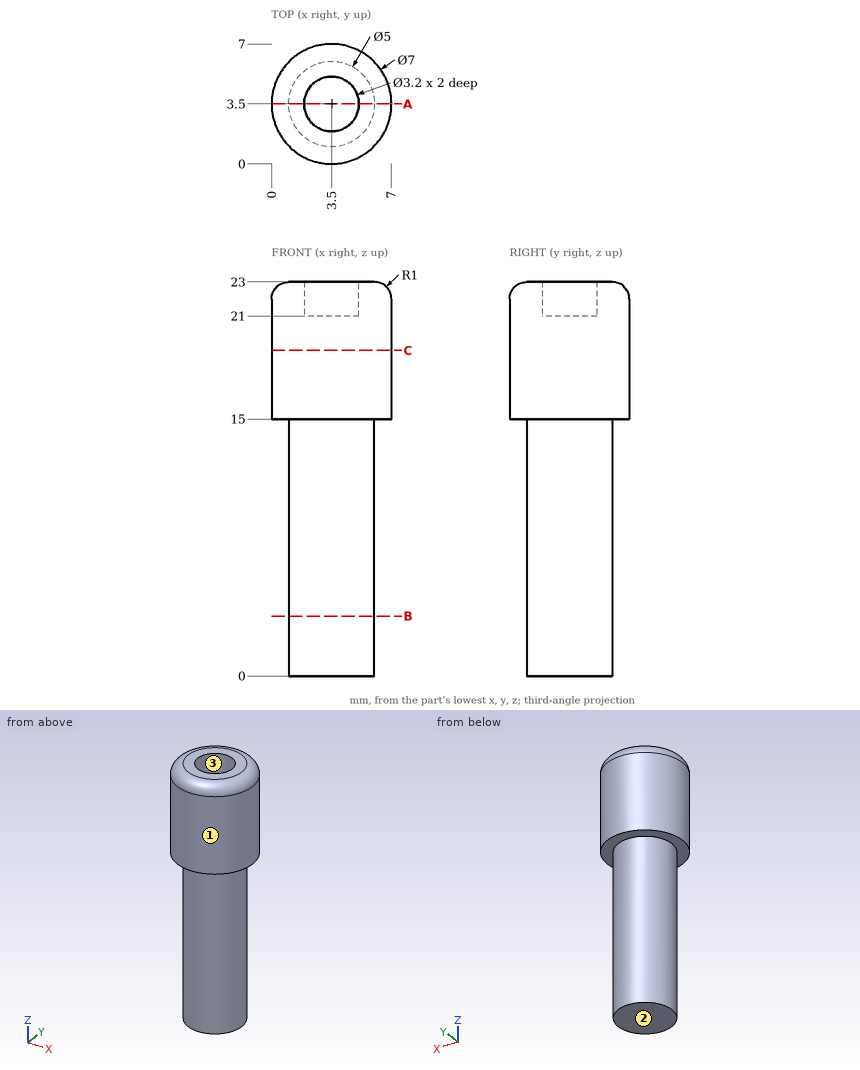
The figure shows three views and two pictorial views of one solid part (mm, origin at its lowest corner). Answer the questions. Round coordinates to 2 decimals unless told otherwise and drop trailing zeros. Order: outer loops, then holes, each group sorted by start corner. A loop starts at its lowest first (then second) coordinate and runs counter-clockwise, first axis right, second up. Notation, with made-up numbers: (89.5, 64.25) - (139.5, 64.25) arc R5 ccw to (139.5, 72.25) - close; hole circle Ø1 at (52, 30). An arc over 180 degrees is marked (long way). Write item = value, one per line. Start each with the question number.
1) Straight lines are drawn through the part: L1, parallel to Y at x = 3.5, z = 22.05; L2, parallel to Y at x = 3.5, z = 22.45; L3, parallel to Z at x = 4.5, y = 3.75. For each, find the intervals that lie inside material, in ascending order.
2) Section B-B, the plane z = 3.5 is taken. Write down the section's boundary in (x, y), plus the area to 3 significant figures.
3) Section A-A, the plane y = 3.5 is taken. Write down the section's boundary in (x, z), plus the area to 3 significant figures.
4) For a pull along X with two mould halves and no side action, classify the marked faces 1, 2 and 3 as released by +X, released by -X, zero draft, split by the parting line, or undercut.
5) Section C-C, the plane z = 19 is taken. Write down the section's boundary in (x, y), plus the area to 3 significant figures.
6) Given pin 1 (1 mm diameter, centred on x = 3, y = 4, fed in from +Z); pin 2 (1 mm diameter, centred on y = 3, z = 4.5, fed in from -X); pin 3 (2 mm diameter, centred on y = 5, z = 16, fed in from -X), each flat-ended and moving along its own axis, determine where each tip first touches the part or whether it passes through.
Results list:
q1.L1 = 0 to 1.9, 5.1 to 7
q1.L2 = 0.11 to 1.9, 5.1 to 6.89
q1.L3 = 0 to 21
q2.outline = circle Ø5 at (3.5, 3.5)
q2.area = 19.6 mm^2
q3.outline = (0, 15) - (1, 15) - (1, 0) - (6, 0) - (6, 15) - (7, 15) - (7, 22) arc R1 ccw to (6, 23) - (5.1, 23) - (5.1, 21) - (1.9, 21) - (1.9, 23) - (1, 23) arc R1 ccw to (0, 22) - close
q3.area = 124 mm^2
q4.face_1 = split by the parting line
q4.face_2 = zero draft
q4.face_3 = undercut
q5.outline = circle Ø7 at (3.5, 3.5)
q5.area = 38.5 mm^2
q6.pin_1 = 21
q6.pin_2 = 1
q6.pin_3 = 0.04
